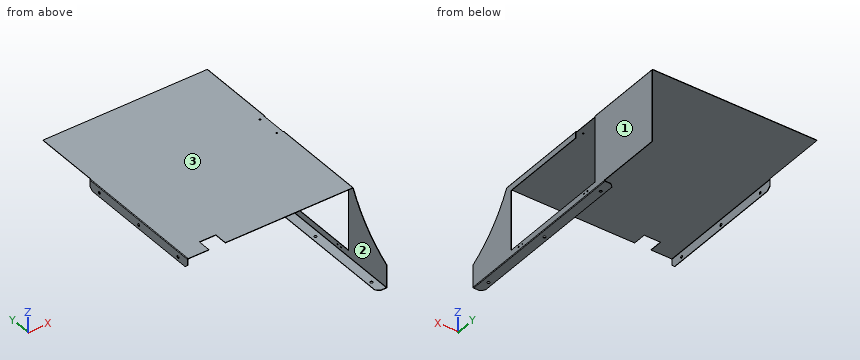
from build123d import *

# Parameters (mm, degrees)
SKETCH_1_W                       = 505
SKETCH_1_H                       = 750
SM_BASE_FLANGE_1_DEPTH           = 1.2
SM_EDGE_FLANGE_1_STRIP_W         = 6.2732
SM_EDGE_FLANGE_1_STRIP_H         = 1.2
SM_EDGE_FLANGE_1_STRIP_CUT_DEPTH = 750
SM_EDGE_FLANGE_1_DEPTH           = 750
CUT_EXTRUDE_1_DEPTH              = 932.264731427
SM_EDGE_FLANGE_2_STRIP_W         = 6.2732
SM_EDGE_FLANGE_2_STRIP_H         = 1.2
SM_EDGE_FLANGE_2_STRIP_CUT_DEPTH = 750
SM_EDGE_FLANGE_2_DEPTH           = 750
SM_EDGE_FLANGE_3_STRIP_W         = 6.2732
SM_EDGE_FLANGE_3_STRIP_H         = 1.2
SM_EDGE_FLANGE_3_STRIP_CUT_DEPTH = 609.290401588
SM_EDGE_FLANGE_3_DEPTH           = 609.290401588
SKETCH_16_W                      = 41.475289024
SKETCH_16_H                      = 200
CUT_EXTRUDE_2_DEPTH              = 932.264731427
SKETCH_17_W                      = 35.547342431
SKETCH_17_H                      = 200
CUT_EXTRUDE_3_DEPTH              = 932.264731427
CHAMFER_1_SIZE                   = 10
SKETCH_19_W                      = 183
SKETCH_19_H                      = 350
CUT_EXTRUDE_4_DEPTH              = 10
SKETCH_20_W                      = 20
SKETCH_20_H                      = 80
CUT_EXTRUDE_5_DEPTH              = 3
CUT_EXTRUDE_6_REACH              = 933.265
SKETCH_21_R                      = 2.5
CUT_EXTRUDE_7_REACH              = 933.265
SKETCH_22_R                      = 2
SKETCH_23_R                      = 4
CUT_EXTRUDE_8_DEPTH              = 10
CUT_EXTRUDE_9_REACH              = 933.265
SKETCH_24_R                      = 4
SKETCH_25_W                      = 50
SKETCH_25_H                      = 40
CUT_EXTRUDE_10_DEPTH             = 10


# Sheet-metal steps are written as plain solids
with BuildPart() as part:
    # Sketch 1 → Базовая кромка1 (new body)
    with BuildSketch(Plane.XY):
        with Locations((252.5, 375)):
            Rectangle(SKETCH_1_W, SKETCH_1_H)
    extrude(amount=-SM_BASE_FLANGE_1_DEPTH)

    # Ребро-кромка1 strip (across the edge) → Ребро-кромка1 strip cut (cut)
    with BuildSketch(Plane(origin=(505, 750, -1.2), x_dir=(-1, 0, 0), z_dir=(0, -1, 0))):
        with Locations((-1.2, -0.6)):
            Rectangle(SM_EDGE_FLANGE_1_STRIP_W, SM_EDGE_FLANGE_1_STRIP_H)
    extrude(amount=SM_EDGE_FLANGE_1_STRIP_CUT_DEPTH, mode=Mode.SUBTRACT)

    # Ребро-кромка1 section (across the edge) → Ребро-кромка1 (add)
    with BuildSketch(Plane(origin=(505, 750, -1.2), x_dir=(-1, 0, 0), z_dir=(0, -1, 0))):
        with BuildLine():
            Line((0, 0.7366), (0, 221.8))
            Line((0, 221.8), (1.2, 221.8))
            Line((1.2, 221.8), (1.2, 0.7366))
            ThreePointArc((1.2, 0.7366), (1.415745145, 0.215745145), (1.9366, 0))
            Line((1.9366, 0), (1.9366, -1.2))
            ThreePointArc((1.9366, -1.2), (0.567217008, -0.632782992), (0, 0.7366))
        make_face()
    extrude(amount=SM_EDGE_FLANGE_1_DEPTH)

    # Эскиз9 → Вырез-Вытянуть1 (cut, through all)
    with BuildSketch(Plane(origin=(505, 0, 0), x_dir=(0, 0, -1), z_dir=(1, 0, 0))):
        with BuildLine():
            Line((1.9366, 140.709598412), (-18.72453306, 140.709598412))
            Line((-18.72453306, 140.709598412), (-18.72453306, 150.079036589))
            ThreePointArc((-18.72453306, 150.079036589), (-305.67985666, -510.169358417), (1.9366, 140.709598412))
        make_face()
    extrude(amount=-CUT_EXTRUDE_1_DEPTH, mode=Mode.SUBTRACT)

    # Ребро-кромка2 strip (across the edge) → Ребро-кромка2 strip cut (cut)
    with BuildSketch(Plane(origin=(503.8, 750, -223), x_dir=(0, 0, 1), z_dir=(0, -1, 0))):
        with Locations((-1.2, -0.6)):
            Rectangle(SM_EDGE_FLANGE_2_STRIP_W, SM_EDGE_FLANGE_2_STRIP_H)
    extrude(amount=SM_EDGE_FLANGE_2_STRIP_CUT_DEPTH, mode=Mode.SUBTRACT)

    # Ребро-кромка2 section (across the edge) → Ребро-кромка2 (add)
    with BuildSketch(Plane(origin=(503.8, 750, -223), x_dir=(0, 0, 1), z_dir=(0, -1, 0))):
        with BuildLine():
            Line((0, 0.7366), (0, 28.8))
            Line((0, 28.8), (1.2, 28.8))
            Line((1.2, 28.8), (1.2, 0.7366))
            ThreePointArc((1.2, 0.7366), (1.415745145, 0.215745145), (1.9366, 0))
            Line((1.9366, 0), (1.9366, -1.2))
            ThreePointArc((1.9366, -1.2), (0.567217008, -0.632782992), (0, 0.7366))
        make_face()
    extrude(amount=SM_EDGE_FLANGE_2_DEPTH)

    # Ребро-кромка3 strip (across the edge) → Ребро-кромка3 strip cut (cut)
    with BuildSketch(Plane(origin=(0, 140.709598412, -1.2), x_dir=(1, 0, 0), z_dir=(0, 1, 0))):
        with Locations((-1.2, -0.6)):
            Rectangle(SM_EDGE_FLANGE_3_STRIP_W, SM_EDGE_FLANGE_3_STRIP_H)
    extrude(amount=SM_EDGE_FLANGE_3_STRIP_CUT_DEPTH, mode=Mode.SUBTRACT)

    # Ребро-кромка3 section (across the edge) → Ребро-кромка3 (add)
    with BuildSketch(Plane(origin=(0, 140.709598412, -1.2), x_dir=(1, 0, 0), z_dir=(0, 1, 0))):
        with BuildLine():
            Line((0, 0.7366), (0, 28.8))
            Line((0, 28.8), (1.2, 28.8))
            Line((1.2, 28.8), (1.2, 0.7366))
            ThreePointArc((1.2, 0.7366), (1.415745145, 0.215745145), (1.9366, 0))
            Line((1.9366, 0), (1.9366, -1.2))
            ThreePointArc((1.9366, -1.2), (0.567217008, -0.632782992), (0, 0.7366))
        make_face()
    extrude(amount=SM_EDGE_FLANGE_3_DEPTH)

    # Эскиз16 → Вырез-Вытянуть2 (cut, through all)
    with BuildSketch(Plane(origin=(505, 0, 0), x_dir=(0, 0, -1), z_dir=(1, 0, 0))):
        with Locations((240.737644512, 650)):
            Rectangle(SKETCH_16_W, SKETCH_16_H)
    extrude(amount=-CUT_EXTRUDE_2_DEPTH, mode=Mode.SUBTRACT)

    # Эскиз17 → Вырез-Вытянуть3 (cut, through all)
    with BuildSketch(Plane.XY):
        with Locations((-14.773671216, 650)):
            Rectangle(SKETCH_17_W, SKETCH_17_H)
    extrude(amount=-CUT_EXTRUDE_3_DEPTH, mode=Mode.SUBTRACT)

    # Фаска1
    chamfer_1_edges = [part.edges().sort_by_distance(p)[0] for p in [
        (0.6, 140.709598412, -30),
        (475, 550, -222.4),
        (0.6, 550, -30),
        (475, 0, -222.4),
    ]]
    chamfer(chamfer_1_edges, length=CHAMFER_1_SIZE)

    # Эскиз19 → Вырез-Вытянуть4 (cut)
    with BuildSketch(Plane(origin=(505, 0, 0), x_dir=(0, 0, -1), z_dir=(1, 0, 0))):
        with Locations((111.5, 335)):
            Rectangle(SKETCH_19_W, SKETCH_19_H)
    extrude(amount=-CUT_EXTRUDE_4_DEPTH, mode=Mode.SUBTRACT)

    # Эскиз20 → Вырез-Вытянуть5 (cut)
    with BuildSketch(Plane(origin=(505, 0, 0), x_dir=(0, 0, -1), z_dir=(1, 0, 0))):
        with Locations((10, 470)):
            Rectangle(SKETCH_20_W, SKETCH_20_H)
    extrude(amount=-CUT_EXTRUDE_5_DEPTH, mode=Mode.SUBTRACT)

    # Эскиз21 → Вырез-Вытянуть6 (cut, up to next)
    with BuildSketch(Plane.XY, mode=Mode.PRIVATE) as cut_extrude_6_sk1:
        with Locations((485.7, 505)):
            Circle(SKETCH_21_R)
    cut_extrude_6_tool1 = extrude(cut_extrude_6_sk1.sketch, amount=-CUT_EXTRUDE_6_REACH, mode=Mode.PRIVATE) & part.part
    # Эскиз21 → Вырез-Вытянуть6 (cut, up to next)
    with BuildSketch(Plane.XY, mode=Mode.PRIVATE) as cut_extrude_6_sk2:
        with Locations((485.7, 435)):
            Circle(SKETCH_21_R)
    cut_extrude_6_tool2 = extrude(cut_extrude_6_sk2.sketch, amount=-CUT_EXTRUDE_6_REACH, mode=Mode.PRIVATE) & part.part
    add(cut_extrude_6_tool1.solids().sort_by_distance((485.7, 505, 0))[0], mode=Mode.SUBTRACT)
    add(cut_extrude_6_tool2.solids().sort_by_distance((485.7, 435, 0))[0], mode=Mode.SUBTRACT)

    # Эскиз22 → Вырез-Вытянуть7 (cut, up to next)
    with BuildSketch(Plane(origin=(505, 0, 0), x_dir=(0, 0, -1), z_dir=(1, 0, 0)), mode=Mode.PRIVATE) as cut_extrude_7_sk1:
        with Locations((211.5, 479)):
            Circle(SKETCH_22_R)
    cut_extrude_7_tool1 = extrude(cut_extrude_7_sk1.sketch, amount=-CUT_EXTRUDE_7_REACH, mode=Mode.PRIVATE) & part.part
    # Эскиз22 → Вырез-Вытянуть7 (cut, up to next)
    with BuildSketch(Plane(origin=(505, 0, 0), x_dir=(0, 0, -1), z_dir=(1, 0, 0)), mode=Mode.PRIVATE) as cut_extrude_7_sk2:
        with Locations((211.5, 464)):
            Circle(SKETCH_22_R)
    cut_extrude_7_tool2 = extrude(cut_extrude_7_sk2.sketch, amount=-CUT_EXTRUDE_7_REACH, mode=Mode.PRIVATE) & part.part
    # Эскиз22 → Вырез-Вытянуть7 (cut, up to next)
    with BuildSketch(Plane(origin=(505, 0, 0), x_dir=(0, 0, -1), z_dir=(1, 0, 0)), mode=Mode.PRIVATE) as cut_extrude_7_sk3:
        with Locations((211.5, 206)):
            Circle(SKETCH_22_R)
    cut_extrude_7_tool3 = extrude(cut_extrude_7_sk3.sketch, amount=-CUT_EXTRUDE_7_REACH, mode=Mode.PRIVATE) & part.part
    # Эскиз22 → Вырез-Вытянуть7 (cut, up to next)
    with BuildSketch(Plane(origin=(505, 0, 0), x_dir=(0, 0, -1), z_dir=(1, 0, 0)), mode=Mode.PRIVATE) as cut_extrude_7_sk4:
        with Locations((211.5, 191)):
            Circle(SKETCH_22_R)
    cut_extrude_7_tool4 = extrude(cut_extrude_7_sk4.sketch, amount=-CUT_EXTRUDE_7_REACH, mode=Mode.PRIVATE) & part.part
    add(cut_extrude_7_tool1.solids().sort_by_distance((505, 479, -211.5))[0], mode=Mode.SUBTRACT)
    add(cut_extrude_7_tool2.solids().sort_by_distance((505, 464, -211.5))[0], mode=Mode.SUBTRACT)
    add(cut_extrude_7_tool3.solids().sort_by_distance((505, 206, -211.5))[0], mode=Mode.SUBTRACT)
    add(cut_extrude_7_tool4.solids().sort_by_distance((505, 191, -211.5))[0], mode=Mode.SUBTRACT)

    # Эскиз23 → Вырез-Вытянуть8 (cut)
    with BuildSketch(Plane(origin=(0, 0, -223), x_dir=(-1, 0, 0), z_dir=(0, 0, -1))):
        with Locations((-487, 510)):
            Circle(SKETCH_23_R)
        with Locations((-487, 275)):
            Circle(SKETCH_23_R)
        with Locations((-487, 40)):
            Circle(SKETCH_23_R)
    extrude(amount=-CUT_EXTRUDE_8_DEPTH, mode=Mode.SUBTRACT)

    # Эскиз24 → Вырез-Вытянуть9 (cut, up to next)
    with BuildSketch(Plane.ZY, mode=Mode.PRIVATE) as cut_extrude_9_sk1:
        with Locations((-18, 510)):
            Circle(SKETCH_24_R)
    cut_extrude_9_tool1 = extrude(cut_extrude_9_sk1.sketch, amount=-CUT_EXTRUDE_9_REACH, mode=Mode.PRIVATE) & part.part
    # Эскиз24 → Вырез-Вытянуть9 (cut, up to next)
    with BuildSketch(Plane.ZY, mode=Mode.PRIVATE) as cut_extrude_9_sk2:
        with Locations((-18, 345.354799206)):
            Circle(SKETCH_24_R)
    cut_extrude_9_tool2 = extrude(cut_extrude_9_sk2.sketch, amount=-CUT_EXTRUDE_9_REACH, mode=Mode.PRIVATE) & part.part
    # Эскиз24 → Вырез-Вытянуть9 (cut, up to next)
    with BuildSketch(Plane.ZY, mode=Mode.PRIVATE) as cut_extrude_9_sk3:
        with Locations((-18, 180.709598412)):
            Circle(SKETCH_24_R)
    cut_extrude_9_tool3 = extrude(cut_extrude_9_sk3.sketch, amount=-CUT_EXTRUDE_9_REACH, mode=Mode.PRIVATE) & part.part
    add(cut_extrude_9_tool1.solids().sort_by_distance((0, 510, -18))[0], mode=Mode.SUBTRACT)
    add(cut_extrude_9_tool2.solids().sort_by_distance((0, 345.354799, -18))[0], mode=Mode.SUBTRACT)
    add(cut_extrude_9_tool3.solids().sort_by_distance((0, 180.709598, -18))[0], mode=Mode.SUBTRACT)

    # Эскиз25 → Вырез-Вытянуть10 (cut)
    with BuildSketch(Plane.XY):
        with Locations((90, 160.709598412)):
            Rectangle(SKETCH_25_W, SKETCH_25_H)
    extrude(amount=-CUT_EXTRUDE_10_DEPTH, mode=Mode.SUBTRACT)


solid = part.part
Here's how the part is built. I have some questions about the finished solid (model axes, mm). Face numbers are marked on the shaded views. Coordinates: 2 decimals unless noted, no trailing zeros. Write each loop counter-clockwise with the first axis right and the second up, starting at its lowest first coordinate (ties: lowest second). Pieces come first, ordered by that corner, then holes.
Item 1: I want a section at A-A on z = -188. Write out the boundary of the cut face in (x, y), and give its area (3 significant figures).
Item 2: I want a section at B-B on y = 664.5. Write out the boundary of the cut face in (x, z), and give its area (3 significant figures).
Item 3: If we mould it in two halves opening along Z, with no side actions, what happens to the marked faces 1, 2 and 3? For each: +Z half, -Z half, draft (parallel to the pull), parting line (faces both ways), or undercut.
Item 4: I want a section at C-C on x = 102. Write out the boundary of the cut face in (y, z).
Item 5: If I drill on line 1 (Y direction, x = 487, z = -222); line 2 (Y direction, x = 504.05, z = -211.5); line 3 (Z direction, x = 482.5, y = 496.5), over which ranges is the centre line in solid material (lowest first)?
Item 6: Will these pins go through, and if not, where does the flat tip stop? pin 1 (1 mm diameter, centred on x = 504, y = 639, fed in from -Z); pin 2 (2.5 mm diameter, centred on y = 479, z = -211.5, fed in from -X); pin 3 (8 mm diameter, centred on y = 602.5, z = -162, fed in from -X); pin 4 (1.5 mm diameter, centred on x = 428, y = 665.5, fed in from -Z).
Item 7: I want a section at D-D on z = -54. Write out the boundary of the cut face in (x, y), and give its area (3 significant figures).
Findings below:
1. outline: (503.8, 0) - (505, 0) - (505, 160) - (503.8, 160) - close; (503.8, 510) - (505, 510) - (505, 750) - (503.8, 750) - close
1. area: 480 mm2
2. outline: (3, -1.2) - (503.06, -1.2) arc R0.74 cw to (503.8, -1.94) - (503.8, -220) - (505, -220) - (505, -1.94) arc R1.94 ccw to (503.06, 0) - (3, 0) - close
2. area: 864 mm2
3. face 1: draft
3. face 2: undercut
3. face 3: +Z half
4. outline: (180.71, -1.2) - (750, -1.2) - (750, 0) - (180.71, 0) - close
5. line 1: y = 0 to 36, 44 to 271, 279 to 506, 514 to 550
5. line 2: y = 0 to 189, 193 to 204, 208 to 462, 466 to 477, 481 to 750
5. line 3: z = -223 to -221.8, -1.2 to 0
6. pin 1: stops at z = -220
6. pin 2: passes through
6. pin 3: stops at x = 503.8
6. pin 4: stops at z = -1.2
7. outline: (503.8, 109.38) - (505, 109.38) - (505, 160) - (503.8, 160) - close; (503.8, 510) - (505, 510) - (505, 750) - (503.8, 750) - close
7. area: 349 mm2
